Input: part model. Units: mm. Frame: model coordinates. Face numbers are marked on the shaded views. A direction names the side the tool comes from. Coordinates: 2 decimals unless noted, no trailing zeros. Order: outer loops, then holes, each group sorted by start corner. A loop starts at its lowest first (then second) coordinate and runs counter-clockwise, first axis right, second up.
from build123d import *

# Parameters (mm, degrees)
SKETCH1_W           = 30
SKETCH1_H           = 28
BOSS_EXTRUDE1_DEPTH = 25
SKETCH2_R           = 11.75
CUT_EXTRUDE1_DEPTH  = 42.484937025
CUT_EXTRUDE2_DEPTH  = 12.5


with BuildPart() as part:
    # Sketch1 → Boss-Extrude1 (new body)
    with BuildSketch(Plane(origin=(0, 0, 0), x_dir=(1, 0, 0), z_dir=(0, 1, 0))):
        Rectangle(SKETCH1_W, SKETCH1_H)
    extrude(amount=BOSS_EXTRUDE1_DEPTH)

    # Sketch2 → Cut-Extrude1 (cut, through all)
    with BuildSketch(Plane.ZY.offset(15)):
        with Locations((0, 12.5)):
            Circle(SKETCH2_R)
    extrude(amount=-CUT_EXTRUDE1_DEPTH, mode=Mode.SUBTRACT)

    # Sketch3 → Cut-Extrude2 (cut)
    with BuildSketch(Plane.XY.offset(14)):
        with BuildLine():
            Line((0, 24.25), (-15, 24.25))
            Line((-15, 24.25), (-15, 0.75))
            Line((-15, 0.75), (0, 0.75))
            ThreePointArc((0, 0.75), (11.75, 12.5), (0, 24.25))
        make_face()
    extrude(amount=-CUT_EXTRUDE2_DEPTH, mode=Mode.SUBTRACT)


solid = part.part
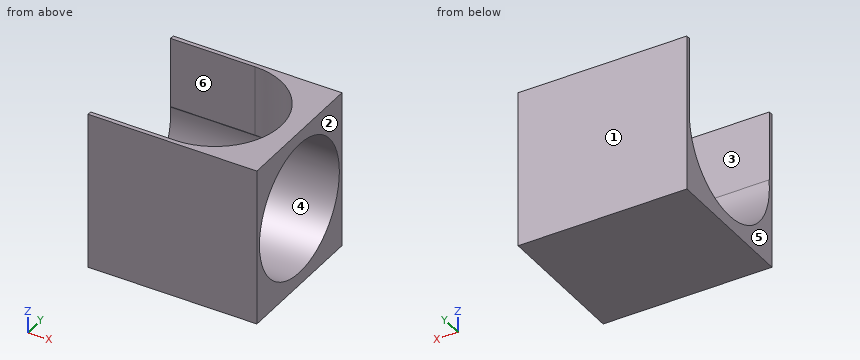
Item 1: Cut plane D-D on x = -11.5. Return loops of the section in (y, z).
Response values:
outline: (0, -14) - (25, -14) - (25, 14) - (24.25, 14) - (24.25, 1.5) - (24.15, 1.5) arc R11.75 cw (long way) to (0.85, 1.5) - (0.75, 1.5) - (0.75, 14) - (0, 14) - close
Item 2: Access query for the marked faces 5 and 6. Directions: +Z, -Z, +X, -X, +Y, -Y. A direction counts if a zero-diameter tool reaches every point of the face in a straight line with its end or side. Return the directions, or none.
Response values:
face 5: +Z, -Z, -X, +Y, -Y
face 6: +Z, -X
Item 3: Pin query (flat end, axial travel): pin 1 Ø2 at (x, y) = (-10, 17.5) entering from +Z; pin 2 Ø10 at (x, y) = (-10.5, 15.5) entering from +Z; pin 3 Ø1 at (x, y) = (-8, 15.5) entering from +Z. Return the tip coordinate at first contact, or that it passes through.
Response values:
pin 1: stops at z = -10.1
pin 2: stops at z = -8.61
pin 3: stops at z = -11.22
Item 4: Cut plane C-C on x = 12.5. Return loops of the section in (y, z), then the cut area to 3 significant figures.
Response values:
outline: (0, -14) - (25, -14) - (25, 14) - (0, 14) - close; hole circle Ø23.5 at (12.5, 0)
area: 266 mm2
Item 5: Cut plane A-A on y = 12.5. Return loops of the section in (x, z), then the cut area to 3 significant figures.
Response values:
outline: (-15, -14) - (15, -14) - (15, -11.75) - (-15, -11.75) - close; (11.75, 11.75) - (15, 11.75) - (15, 14) - (11.75, 14) - close
area: 74.8 mm2
Item 6: Cut plane B-B on z = 0. Return loops of the section in (x, y), then the cut area to 3 significant figures.
Response values:
outline: (-15, 0) - (15, 0) - (15, 0.75) - (-15, 0.75) - close; (-15, 24.25) - (15, 24.25) - (15, 25) - (-15, 25) - close
area: 45.0 mm2
Item 7: Ray query, probe 1 along Y at (x, z) = (-1.5, 0); probe 2 along Z at (x, y) = (12.75, 18.5); probe 3 along Y at (x, z) = (5, 6.75). Return the intervals inside material, ascending.
Response values:
probe 1: y = 0 to 0.75, 24.25 to 25
probe 2: z = -14 to -10.1, 10.1 to 14
probe 3: y = 0 to 1.87, 23.13 to 25
Item 8: Draft query along Y for the marked faces 1, 2, 3 and 4. Return one class per face: pulls with the +Y half, pulls with the -Y half, needs draft (parallel to the pull), parting line crosses it, or undercut.
Response values:
face 1: pulls with the +Y half
face 2: needs draft
face 3: undercut
face 4: undercut
